Input: part model. Units: mm. Frame: model coordinates. A direction names the side the tool comes from. Round coordinates to 2 decimals unless told otherwise and drop trailing zeros. Write each loop counter-clockwise with the first axis right and the second up, starting at its lowest first coordinate (ties: lowest second). Pieces come first, ordered by that corner, then holes. Notation, with made-up numbers: (12.5, 1) -> (32.5, 1) arc R19 ccw to (32.5, 10) -> close; hole circle Ø1 at (63, -1.75). An arc over 180 degrees is marked (long way). Write item = value, one per line. Start each with the question number.
Autodesk Inventor part; units mm, degrees
ref_plane "YZ Plane" through (0, 0, 0) normal (1, 0, 0) x (0, 1, 0)
ref_plane "XZ Plane" through (0, 0, 0) normal (0, 1, 0) x (-1, 0, 0)
sketch "Sketch1" plane through (0, 0, 0) normal (0, 1, 0) x (-1, 0, 0)
  line L0 (139.7, 12.7) -> (-139.7, 12.7)
  line L1 (-139.7, 12.7) -> (-139.7, -12.7)
  line L2 (-139.7, -12.7) -> (139.7, -12.7)
  line L3 (139.7, -12.7) -> (139.7, 12.7)
  line L4 (139.7, 12.7) -> (-139.7, -12.7) construction
  line L5 (-139.7, 12.7) -> (139.7, -12.7) construction
  point P0 (0, 0)
  dimension "d0" = 279.4
  dimension "d1" = 25.4
extrude "Extrusion1" add sketch "Sketch1" along normal mid plane 25.4
sketch "Sketch3" plane through (0, 12.7, 0) normal (0, 1, 0) x (1, 0, 0)
  line L0 (-139.7, -6.858) -> (76.2, -6.858)
  line L1 (76.2, -6.858) -> (76.2, 6.858)
  line L2 (76.2, 6.858) -> (-139.7, 6.858)
  line L3 (-139.7, 6.858) -> (-139.7, -6.858)
  line L4 (-139.7, -6.858) -> (76.2, 6.858) construction
  line L5 (76.2, -6.858) -> (-139.7, 6.858) construction
  line L6 (-139.7, 12.7) -> (-139.7, -12.7)
  point P0 (0, 0)
  point P1 (-31.75, 0)
  dimension "d7" = 0
  dimension "d8" = 13.716
  dimension "d9" = 215.9
extrude "Extrusion2" cut sketch "Sketch3" against normal through all
sketch "Sketch4" plane through (0, 12.7, 0) normal (0, 1, 0) x (1, 0, 0)
  line L0 (139.7, 12.7) -> (-139.7, 12.7)
  line L1 (139.7, 12.7) -> (101.6, 12.7)
  line L2 (101.6, 12.7) -> (101.6, 6.35)
  line L3 (101.6, 6.35) -> (139.7, 6.35)
  line L4 (139.7, 6.35) -> (139.7, 12.7)
  line L5 (139.7, 0) -> (76.2, 0) construction
  line L6 (76.2, 6.858) -> (76.2, -6.858) construction
  point P0 (0, 0)
  point P1 (101.6, 12.7)
  dimension "d12" = 38.1
  dimension "d13" = 6.35
extrude "Extrusion3" cut sketch "Sketch4" against normal through all
mirror "Mirror1" about plane through (0, 0, 0) normal (0, 0, 1) of "Extrusion3"
sketch "Sketch5" plane through (-139.7, -12.7, 12.7) normal (0, 0, 1) x (1, 0, 0)
  circle A0 centre (12.7, 12.7) radius 5.2705
  circle A1 centre (266.7, 12.7) radius 5.2705
  line L0 (0, 0) -> (0, 25.4)
  line L1 (279.4, 25.4) -> (279.4, 0)
  point P0 (139.7, 12.7)
  dimension "d16" = 10.541
  dimension "d17" = 12.7
  dimension "d18" = 12.7
extrude "Extrusion4" cut sketch "Sketch5" against normal through all
sketch "Sketch6" plane through (0, 12.7, 0) normal (0, 1, 0) x (1, 0, 0)
  line L0 (-139.7, -12.7) -> (101.6, -12.7)
  line L1 (-139.7, 12.3621) -> (-136.525, 12.3621)
  line L2 (-136.525, 12.3621) -> (-136.525, -12.7)
  line L3 (-136.525, -12.7) -> (-139.7, -12.7)
  line L4 (-139.7, -12.7) -> (-139.7, 12.3621)
  line L5 (139.7, 6.35) -> (101.6, 6.35)
  line L6 (101.6, -6.35) -> (139.7, -6.35)
  line L7 (139.7, 6.35) -> (136.525, 6.35)
  line L8 (136.525, 6.35) -> (136.525, -6.35)
  line L9 (136.525, -6.35) -> (139.7, -6.35)
  line L10 (139.7, -6.35) -> (139.7, 6.35)
  point P0 (0, 0)
  dimension "d21" = 3.175
  dimension "d22" = 3.175
extrude "Extrusion5" cut sketch "Sketch6" against normal through all
properties part number "connectingRodV03-7-in" material "PET Plastic"
1. Section D-D (z = 4). Output: boundary loops of the cut face in (x, y) (1 decimal), then the cut area to 3 significant figures.
2. Reachability of faces 4 (the flat face through (119, 0, -6.35)), 5 (the flat face through (101.6, 0, 9)), 6 (the flat face through (-136.525, 0, 10)) from +Z, -Z, +X, -X, +Y, -Y: full face, straight path, thin tool, end or side. Return the list, or none.
3. Mould query, pull axis Y, two halves, no side actions, for faces 1 (the cylindrical face through (-132.265, 0.232, -9.738)), 2 (the flat face through (-32, 0, 6.858)), 3 (the flat face through (0, 12.7, 9)). Classes: pulls with the +Y half, pulls with the -Y half, needs draft (parallel to the pull), parting line crosses it, or undercut.
4. Pin query (flat end, axial travel): P1, Ø12.5, axis at x = 121.5, y = -3, coming from the +Z side; P2, Ø1.6, axis at x = -138, y = -6, coming from the +Z side; P3, Ø13.5, axis at x = 127, y = 0, coming from the -Z side; P4, Ø9.5, axis at x = -127, y = 0, coming from the +Z side. Return the tip coordinate at first contact, or that it passes through.
5. Line query: line 1 along Z through (x, y) = (72.5, -7); line 2 along Y through (x, z) = (-127, -8); line 3 along X through (y, z) = (-8.5, 2.75) (3 decimals). Output: solid intervals per line, ascending.
6. Section A-A (x = -77). Output: boundary loops of the cut face in (y, z).
7. Section C-C (y = 0). State how many separate pieces and enclosed holes the cut face has, then the cut area to 3 significant figures.
8. Section B-B (x = -127). Output: boundary loops of the cut face in (y, z).
Check sheet entries:
q1.outline = (76.2, -12.7) -> (136.5, -12.7) -> (136.5, 12.7) -> (76.2, 12.7) -> close; hole circle Ø10.5 at (127, 0)
q1.area = 1,440 mm2
q2.face_4 = -Z, +X, +Y, -Y
q2.face_5 = +Z, +X, +Y, -Y
q2.face_6 = +Z, -X, +Y, -Y
q3.face_1 = undercut
q3.face_2 = needs draft
q3.face_3 = pulls with the +Y half
q4.P1 = 6.35
q4.P2 = -12.36
q4.P3 = -6.35
q4.P4 = through
q5.line_1 = -12.7 to -6.86, 6.86 to 12.7
q5.line_2 = -12.7 to -5.27, 5.27 to 12.7
q5.line_3 = 76.2 to 136.525
q6.outline = (-12.7, -12.7) -> (12.7, -12.7) -> (12.7, -6.86) -> (-12.7, -6.86) -> close; (-12.7, 6.86) -> (12.7, 6.86) -> (12.7, 12.7) -> (-12.7, 12.7) -> close
q7.separate_pieces = 4
q7.enclosed_holes = 0
q7.area = 3,320 mm2
q8.outline = (-12.7, -12.7) -> (-5.27, -12.7) -> (-5.27, -6.86) -> (-12.7, -6.86) -> close; (-12.7, 6.86) -> (-5.27, 6.86) -> (-5.27, 12.7) -> (-12.7, 12.7) -> close; (5.27, -12.7) -> (12.7, -12.7) -> (12.7, -6.86) -> (5.27, -6.86) -> close; (5.27, 6.86) -> (12.7, 6.86) -> (12.7, 12.7) -> (5.27, 12.7) -> close
